Geometry: final body of the model. Coordinates: model frame, mm. Coordinates: 2 decimals unless noted, no trailing zeros. Order: outer loops, then holes, each group sorted by start corner. A loop starts at its lowest first (then second) coordinate and runs counter-clockwise, first axis right, second up. Notation, with made-up numbers: (59.25, 76) - (110.25, 76) arc R28 cw to (110.25, 112) - close; hole circle Ø9 at (45.25, -12). An arc over 180 degrees is marked (long way). Use a Markdown table: item, result. Add a question column.
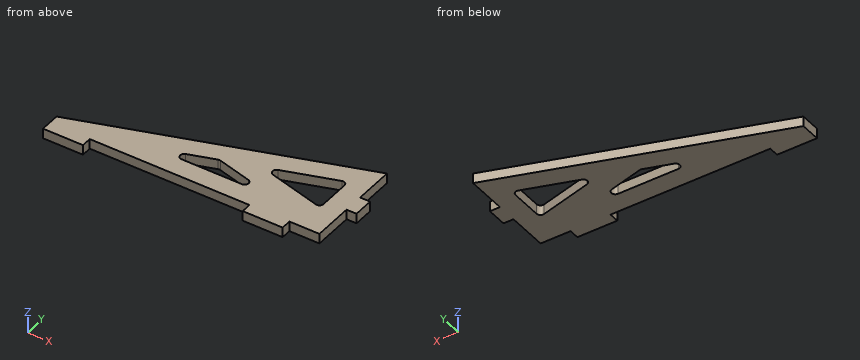
```python
from build123d import *

# Parameters (mm, degrees)
BOSS_EXTRUDE1_DEPTH = 6.35
CUT_EXTRUDE1_DEPTH  = 226.36350526
FILLET1_R           = 2.54


with BuildPart() as part:
    # Sketch2 → Boss-Extrude1 (new body)
    with BuildSketch(Plane.XY):
        Polygon((-92.950015109, 148.30800019), (78.499984891, 205.20400019), (78.499984891, 180.05800019), (84.849984891, 180.05800019), (84.849984891, 167.35800019), (78.499984891, 167.35800019), (78.499984891, 141.95800019), (59.449984891, 141.95800019), (59.449984891, 135.60800019), (34.049984891, 135.60800019), (34.049984891, 141.95800019), (-67.550015109, 141.95800019), (-67.550015109, 135.60800019), (-92.950015109, 135.60800019), (-92.950015109, 141.95800019), align=None)
    extrude(amount=BOSS_EXTRUDE1_DEPTH)

    # Sketch3 → Cut-Extrude1 (cut, through all)
    with BuildSketch(Plane.XY.offset(6.35)):
        Polygon((-1.019446214, 165.434292154), (-33.492647443, 154.65800019), (40.515121465, 154.65800019), align=None)
        Polygon((65.799984891, 187.608444106), (21.169587996, 172.797764247), (65.799984891, 161.218248334), align=None)
    extrude(amount=-CUT_EXTRUDE1_DEPTH, mode=Mode.SUBTRACT)

    # Fillet1
    fillet1_edges = [part.edges().sort_by_distance(p)[0] for p in [
        (65.799984891, 161.218248334, 3.175),
        (21.169587996, 172.797764247, 3.175),
        (65.799984891, 187.608444106, 3.175),
        (40.515121465, 154.65800019, 3.175),
        (-33.492647443, 154.65800019, 3.175),
        (-1.019446214, 165.434292154, 3.175),
    ]]
    fillet(fillet1_edges, radius=FILLET1_R)


solid = part.part
```
1) Section D-D (y = 190). Return loops of the section in (x, z).
2) Section B-B (x = 45). Return loops of the section in (y, z).
3) Pin query (flat end, axial travel): pin 1 (3 mm diameter, centred on x = 80.5, z = 3.5, fed in from -Y); pin 2 (3 mm diameter, centred on y = 152, z = 1.5, fed in from +X); pin 3 (3 mm diameter, centred on x = 64.5, z = 2, fed in from +Y). Return the tip coordinate at first contact, or that it passes through.
4) Section C-C (x = -8). Return loops of the section in (y, z).
5) Section A-A (z = 3). Return loops of the section in (x, y).
6) Ray query, line 1 along X through (y, z) = (141, 0.5); line 2 along Y through (x, z) = (40.5, 0.75); line 3 along Y through (x, z) = (-15, 5). Return the intervals inside material, ascending.
Values follow:
| question | item | result |
|---|---|---|
| 1 | outline | (32.68, 0) - (78.5, 0) - (78.5, 6.35) - (32.68, 6.35) - close |
| 2 | outline | (135.61, 0) - (166.61, 0) - (166.61, 6.35) - (135.61, 6.35) - close; (180.71, 0) - (194.09, 0) - (194.09, 6.35) - (180.71, 6.35) - close |
| 3 | pin 1 | stops at y = 167.36 |
| 3 | pin 2 | stops at x = 78.5 |
| 3 | pin 3 | stops at y = 201.06 |
| 4 | outline | (141.96, 0) - (154.66, 0) - (154.66, 6.35) - (141.96, 6.35) - close; (163.12, 0) - (176.5, 0) - (176.5, 6.35) - (163.12, 6.35) - close |
| 5 | outline | (-92.95, 135.61) - (-67.55, 135.61) - (-67.55, 141.96) - (34.05, 141.96) - (34.05, 135.61) - (59.45, 135.61) - (59.45, 141.96) - (78.5, 141.96) - (78.5, 167.36) - (84.85, 167.36) - (84.85, 180.06) - (78.5, 180.06) - (78.5, 205.2) - (-92.95, 148.31) - close; hole (-18.57, 159.61) arc R2.54 ccw to (-17.77, 154.66) - (20.61, 154.66) arc R2.54 ccw to (21.25, 159.66) - (-0.29, 165.25) arc R2.54 ccw to (-1.73, 165.2) - close; hole (29.33, 175.51) arc R2.54 ccw to (29.5, 170.64) - (62.62, 162.04) arc R2.54 ccw to (65.8, 164.5) - (65.8, 184.09) arc R2.54 ccw to (62.46, 186.5) - close |
| 6 | line 1 | x = -92.95 to -67.55, 34.05 to 59.45 |
| 6 | line 2 | y = 135.61 to 167.78, 179.21 to 192.59 |
| 6 | line 3 | y = 141.96 to 154.66, 160.79 to 174.18 |
